The model under review builds one solid part; all positions refer to its coordinate system, in mm. A direction names the side the tool comes from. Coordinates: 2 decimals unless noted, no trailing zeros. Write each loop counter-clockwise with the first axis right and the second up, starting at its lowest first coordinate (ties: lowest second). Pieces come first, ordered by that corner, then holes. Notation, with made-up numbers: (-12, 27.25) - (-5, 27.25) arc R30 ccw to (-5, 57.25) - close; hole circle Ø7 at (-20.5, 7.5). An arc over 180 degrees is marked (long way). Put each result on its own line as item: value. Start each with the question number.
Item 1: For pin 1 (3.5 mm diameter, centred on x = 0, z = 0, fed in from +Y); pin 2 (1 mm diameter, centred on x = -11, y = 1.5, fed in from -Z); pin 3 (1 mm diameter, centred on y = -0.5, z = -1, fed in from +X), all flat-tipped, find the tip position at first contact; note any pin that passes through.
Item 2: To check wall thickness, follow L1, parallel to Y at x = -1, z = -2; L2, parallel to Z at x = 6.5, y = 0; L3, parallel to Z at x = -16, y = -0.4. State the ranges of each line that lie inside material, in increasing order. Write a range as [from, to].
Item 3: Mouldability with a two-part tool opening along Z and no side actions: class faces 1 (the face through (10.632, -0.016, 0.403)), 2 (the face through (19, 0, 0)), 3 (the face through (-10.52, 0.02, -3.47)), 4 (the face through (-10.744, -0.016, 0.098)) as pulls with the +Z half, pulls with the -Z half, needs draft (parallel to the pull), parting line crosses it, or undercut.
Item 4: Consider section A-A on y = 0.5. State how many separate pieces and enclosed holes the cut face has, then the cut area to 3 significant figures.
Item 5: Machinability: for faces 5 (the face through (-6.71, -0.02, -0.69)), 6 (the face through (1.3, 1.15, 1.2)), which of the approach directions +Z, -Z, +X, -X, +Y, -Y give a long, thin tool a straight path to every point of the face, cutting with its end or side? Answer none if there is none.
Item 6: Consider section C-C on z = 4. Give the boundary of the cut face in (x, y).
Item 7: Consider section B-B on x = -13. Give the boundary of the cut face in (y, z), then the cut area to 3 significant figures.
Item 8: Consider section D-D on x = -7. Give the boundary of the cut face in (y, z).
```python
from build123d import *

# Parameters (mm, degrees)
SKETCH2_R           = 6
SKETCH2_R_2         = 1.5
BOSS_EXTRUDE1_DEPTH = 1.15
SKETCH3_R           = 4.4
BOSS_EXTRUDE2_DEPTH = 3.2
SKETCH4_R           = 0.75
BOSS_EXTRUDE3_DEPTH = 1.15
CIRPATTERN1_COUNT   = 2


with BuildPart() as part:
    # Sketch2 → Boss-Extrude1 (new, symmetric)
    with BuildSketch(Plane(origin=(0, 0, 0), x_dir=(1, 0, 0), z_dir=(0, 1, 0))):
        with Locations(Location((0, 0, 0), (0, 0, 270))):
            Circle(SKETCH2_R)
        with Locations(Location((0, 0, 0), (0, 0, 270))):
            Circle(SKETCH2_R_2, mode=Mode.SUBTRACT)
    extrude(amount=BOSS_EXTRUDE1_DEPTH, both=True)

    # Sketch3 → Boss-Extrude2 (add)
    with BuildSketch(Plane(origin=(0, 1.15, 0), x_dir=(1, 0, 0), z_dir=(0, 1, 0))):
        with Locations(Location((0, 0, 0), (0, 0, 270))):
            Circle(SKETCH3_R)
        with BuildLine():
            Line((0.107421435, 2.898009771), (0.338399731, 2.678709694))
            Line((0.338399731, 2.678709694), (0.61665913, 2.83367809))
            ThreePointArc((0.61665913, 2.83367809), (0.721200673, 2.808891167), (0.824752316, 2.780248841))
            Line((0.824752316, 2.780248841), (0.993936292, 2.510396512))
            Line((0.993936292, 2.510396512), (1.301992734, 2.591295993))
            ThreePointArc((1.301992734, 2.591295993), (1.397085655, 2.541289372), (1.490260976, 2.48779465))
            Line((1.490260976, 2.48779465), (1.587020181, 2.184345885))
            Line((1.587020181, 2.184345885), (1.905517346, 2.186093238))
            ThreePointArc((1.905517346, 2.186093238), (1.985186607, 2.11400902), (2.062131058, 2.039023173))
            Line((2.062131058, 2.039023173), (2.080385755, 1.721044772))
            Line((2.080385755, 1.721044772), (2.389311295, 1.643530205))
            ThreePointArc((2.389311295, 1.643530205), (2.448550984, 1.553897705), (2.504429862, 1.46213237))
            Line((2.504429862, 1.46213237), (2.443033042, 1.149604087))
            Line((2.443033042, 1.149604087), (2.722976028, 0.997698125))
            ThreePointArc((2.722976028, 0.997698125), (2.758063897, 0.896149284), (2.789366126, 0.793370413))
            Line((2.789366126, 0.793370413), (2.652175577, 0.505929549))
            Line((2.652175577, 0.505929549), (2.885546163, 0.289177003))
            ThreePointArc((2.885546163, 0.289177003), (2.894277512, 0.182092507), (2.899036259, 0.074758075))
            Line((2.899036259, 0.074758075), (2.694672167, -0.169534403))
            Line((2.694672167, -0.169534403), (2.866806821, -0.437514174))
            ThreePointArc((2.866806821, -0.437514174), (2.848633027, -0.543405812), (2.826549281, -0.648551587))
            Line((2.826549281, -0.648551587), (2.567852594, -0.834345885))
            Line((2.567852594, -0.834345885), (2.667935462, -1.136714727))
            ThreePointArc((2.667935462, -1.136714727), (2.623998452, -1.234759946), (2.576459817, -1.331110368))
            Line((2.576459817, -1.331110368), (2.279685399, -1.446732346))
            Line((2.279685399, -1.446732346), (2.301427906, -1.764491312))
            ThreePointArc((2.301427906, -1.764491312), (2.234488404, -1.84852957), (2.164481907, -1.930030589))
            Line((2.164481907, -1.930030589), (1.848277186, -1.968215294))
            Line((1.848277186, -1.968215294), (1.790313171, -2.281398419))
            ThreePointArc((1.790313171, -2.281398419), (1.704577232, -2.346149284), (1.616501638, -2.40767989))
            Line((1.616501638, -2.40767989), (1.30073492, -2.366028036))
            Line((1.30073492, -2.366028036), (1.166706475, -2.654956874))
            ThreePointArc((1.166706475, -2.654956874), (1.067561203, -2.696351809), (0.966950626, -2.734045809))
            Line((0.966950626, -2.734045809), (0.671462695, -2.615174535))
            Line((0.671462695, -2.615174535), (0.469791321, -2.861694623))
            ThreePointArc((0.469791321, -2.861694623), (0.363466377, -2.877132634), (0.25664255, -2.888621575))
            Line((0.25664255, -2.888621575), (0, -2.7))
            Line((0, -2.7), (-0.25664255, -2.888621575))
            ThreePointArc((-0.25664255, -2.888621575), (-0.363466377, -2.877132634), (-0.469791321, -2.861694623))
            Line((-0.469791321, -2.861694623), (-0.671462695, -2.615174535))
            Line((-0.671462695, -2.615174535), (-0.966950626, -2.734045809))
            ThreePointArc((-0.966950626, -2.734045809), (-1.067561203, -2.696351809), (-1.166706475, -2.654956874))
            Line((-1.166706475, -2.654956874), (-1.30073492, -2.366028036))
            Line((-1.30073492, -2.366028036), (-1.616501638, -2.40767989))
            ThreePointArc((-1.616501638, -2.40767989), (-1.704577232, -2.346149284), (-1.790313171, -2.281398419))
            Line((-1.790313171, -2.281398419), (-1.848277186, -1.968215294))
            Line((-1.848277186, -1.968215294), (-2.164481907, -1.930030589))
            ThreePointArc((-2.164481907, -1.930030589), (-2.234488404, -1.84852957), (-2.301427906, -1.764491312))
            Line((-2.301427906, -1.764491312), (-2.279685399, -1.446732346))
            Line((-2.279685399, -1.446732346), (-2.576459817, -1.331110368))
            ThreePointArc((-2.576459817, -1.331110368), (-2.623998452, -1.234759946), (-2.667935462, -1.136714727))
            Line((-2.667935462, -1.136714727), (-2.567852594, -0.834345885))
            Line((-2.567852594, -0.834345885), (-2.826549281, -0.648551587))
            ThreePointArc((-2.826549281, -0.648551587), (-2.848633027, -0.543405812), (-2.866806821, -0.437514174))
            Line((-2.866806821, -0.437514174), (-2.694672167, -0.169534403))
            Line((-2.694672167, -0.169534403), (-2.899036259, 0.074758075))
            ThreePointArc((-2.899036259, 0.074758075), (-2.894277512, 0.182092507), (-2.885546163, 0.289177003))
            Line((-2.885546163, 0.289177003), (-2.652175577, 0.505929549))
            Line((-2.652175577, 0.505929549), (-2.789366126, 0.793370413))
            ThreePointArc((-2.789366126, 0.793370413), (-2.758063897, 0.896149284), (-2.722976028, 0.997698125))
            Line((-2.722976028, 0.997698125), (-2.443033042, 1.149604087))
            Line((-2.443033042, 1.149604087), (-2.504429862, 1.46213237))
            ThreePointArc((-2.504429862, 1.46213237), (-2.448550984, 1.553897705), (-2.389311295, 1.643530205))
            Line((-2.389311295, 1.643530205), (-2.080385755, 1.721044772))
            Line((-2.080385755, 1.721044772), (-2.062131058, 2.039023173))
            ThreePointArc((-2.062131058, 2.039023173), (-1.985186607, 2.11400902), (-1.905517346, 2.186093238))
            Line((-1.905517346, 2.186093238), (-1.587020181, 2.184345885))
            Line((-1.587020181, 2.184345885), (-1.490260976, 2.48779465))
            ThreePointArc((-1.490260976, 2.48779465), (-1.397085655, 2.541289372), (-1.301992734, 2.591295993))
            Line((-1.301992734, 2.591295993), (-0.993936292, 2.510396512))
            Line((-0.993936292, 2.510396512), (-0.824752316, 2.780248841))
            ThreePointArc((-0.824752316, 2.780248841), (-0.721200673, 2.808891167), (-0.61665913, 2.83367809))
            Line((-0.61665913, 2.83367809), (-0.338399731, 2.678709694))
            Line((-0.338399731, 2.678709694), (-0.107421435, 2.898009771))
            ThreePointArc((-0.107421435, 2.898009771), (0, 2.9), (0.107421435, 2.898009771))
        make_face(mode=Mode.SUBTRACT)
    extrude(amount=BOSS_EXTRUDE2_DEPTH)

    # Sketch4 → Boss-Extrude3 (add, symmetric)
    with BuildSketch(Plane(origin=(0, 0, 0), x_dir=(1, 0, 0), z_dir=(0, 1, 0))):
        with BuildLine():
            Line((3.968626967, 4.5), (16.888114198, 2.469689731))
            ThreePointArc((16.888114198, 2.469689731), (19, 0), (16.888114198, -2.469689731))
            Line((16.888114198, -2.469689731), (3.968626967, -4.5))
            ThreePointArc((3.968626967, -4.5), (6, 0), (3.968626967, 4.5))
        make_face()
        with Locations(Location((16, 0, 0), (0, 0, 270))):
            Circle(SKETCH4_R, mode=Mode.SUBTRACT)
        with Locations(Location((13, 0, 0), (0, 0, 270))):
            Circle(SKETCH4_R, mode=Mode.SUBTRACT)
        with Locations(Location((10, 0, 0), (0, 0, 270))):
            Circle(SKETCH4_R, mode=Mode.SUBTRACT)
        with Locations(Location((7, 0, 0), (0, 0, 270))):
            Circle(SKETCH4_R, mode=Mode.SUBTRACT)
    boss_extrude3 = extrude(amount=BOSS_EXTRUDE3_DEPTH, both=True)

    # CirPattern1: Boss-Extrude3 ×2 about axis
    cirpattern1_axis = Axis((0, 0, 0), (0, 1, 0))
    for i in range(1, CIRPATTERN1_COUNT):
        add(boss_extrude3.rotate(cirpattern1_axis, i * 360 / CIRPATTERN1_COUNT))


solid = part.part
```
Report:
1. pin 1: y = 1.15
1. pin 2: z = -3.45
1. pin 3: x = 18.95
2. L1: [-1.15, 1.15]
2. L2: [-4.1, -0.56], [0.56, 4.1]
2. L3: [-2.61, -0.75], [0.75, 2.61]
3. face 1: undercut
3. face 2: parting line crosses it
3. face 3: pulls with the -Z half
3. face 4: undercut
4. separate pieces: 1
4. enclosed holes: 9
4. area: 262 mm²
5. face 5: +Y, -Y
5. face 6: +Y
6. outline: (-7.15, -1.15) - (7.15, -1.15) - (7.15, 1.15) - (1.83, 1.15) - (1.83, 4.35) - (-1.83, 4.35) - (-1.83, 1.15) - (-7.15, 1.15) - close
7. outline: (-1.15, -3.08) - (1.15, -3.08) - (1.15, -0.75) - (-1.15, -0.75) - close; (-1.15, 0.75) - (1.15, 0.75) - (1.15, 3.08) - (-1.15, 3.08) - close
7. area: 10.7 mm²
8. outline: (-1.15, -4.02) - (1.15, -4.02) - (1.15, -0.75) - (-1.15, -0.75) - close; (-1.15, 0.75) - (1.15, 0.75) - (1.15, 4.02) - (-1.15, 4.02) - close
